Geometry: final body of the model. Coordinates: model frame, mm. Face numbers are marked on the shaded views. A direction names the side the tool comes from. Round coordinates to 2 decimals unless told otherwise and drop trailing zeros. Write each loop counter-clockwise with the first axis right and the second up, starting at its lowest first coordinate (ties: lowest second). Pieces come first, ordered by that corner, then holes. Notation, with made-up numbers: (-21, -39) -> (26, -39) arc R21 ccw to (26, -32) -> close; hole circle Ø5 at (19, 28). An arc over 180 degrees is marked (long way). Use one line per item in the form item = value. Start each with the question number.
1. Reachability of the marked faces 5, 6, 7 and 8 from +Z, -Z, +X, -X, +Y, -Y: full face, straight path, thin tool, end or side. Return the list, or none.
2. Cut plane B-B, the plane x = -29.5. Return the cut outline in (y, z).
3. Cut plane C-C, the plane z = 195. Return the cut outline in (x, y), plus the area to 3 significant figures.
4. Pin query (flat end, axial travel): pin 1 Ø10 at (x, z) = (12, 231) entering from +Y; pin 2 Ø4 at (x, z) = (33.5, 132.5) entering from +Y; pin 3 Ø25 at (y, z) = (-3, 237.5) entering from +X; pin 4 Ø10 at (x, y) = (-52.5, 21.5) entering from +Z. Return the tip coordinate at first contact, or that it passes through.
5. Cut plane D-D, the plane y = 54.5. Return the cut outline in (x, z), plus the area to 3 significant figures.
6. Line query: L1, parallel to X at y = 11, z = 203; L2, parallel to Y at x = 0, z = 138.5. Output: solid intervals per line, ascending.
7. Cut plane A-A, the plane y = 0. Return the cut outline in (x, z).
8. Draft query along Y for the marked faces 1, 2, 3 and 4. Return one class per face: pulls with the +Y half, pulls with the -Y half, needs draft (parallel to the pull), parting line crosses it, or undercut.
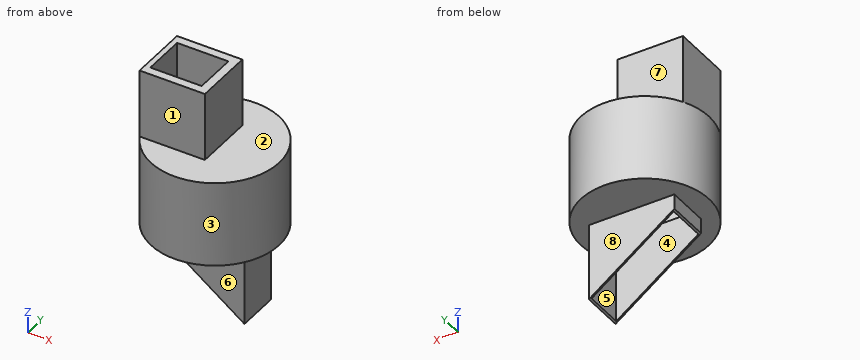
```python
from build123d import *

# Parameters (mm, degrees)
CROQUIS1_W              = 100
CROQUIS1_H              = 50
CROQUIS1_W_2            = 96
CROQUIS1_H_2            = 46
SALIENTE_EXTRUIR1_DEPTH = 100
CORTAR_EXTRUIR1_DEPTH   = 100
CROQUIS3_R              = 75
CROQUIS3_W              = 100
CROQUIS3_H              = 50
SALIENTE_EXTRUIR2_DEPTH = 10
SALIENTE_EXTRUIR3_START = 80
CROQUIS4_R              = 75
CROQUIS4_R_2            = 65
SALIENTE_EXTRUIR3_DEPTH = 80
SALIENTE_EXTRUIR4_START = 10
CROQUIS5_R              = 75
CROQUIS5_W              = 60
CROQUIS5_H              = 50
SALIENTE_EXTRUIR4_DEPTH = 10
CROQUIS6_W              = 76.332495807
CROQUIS6_H              = 70
CROQUIS6_W_2            = 60
CROQUIS6_H_2            = 50
SALIENTE_EXTRUIR5_DEPTH = 80


with BuildPart() as part:
    # Croquis1 → Saliente-Extruir1 (new body)
    with BuildSketch(Plane.XY):
        Rectangle(CROQUIS1_W, CROQUIS1_H)
        Rectangle(CROQUIS1_W_2, CROQUIS1_H_2, mode=Mode.SUBTRACT)
    extrude(amount=SALIENTE_EXTRUIR1_DEPTH)

    # Croquis2 → Cortar-Extruir1 (cut)
    with BuildSketch(Plane(origin=(0, 25, 0), x_dir=(1, 0, 0), z_dir=(0, 1, 0))):
        Polygon((-50, 0), (50, 0), (-50, -72.654252801), align=None)
    extrude(amount=-CORTAR_EXTRUIR1_DEPTH, mode=Mode.SUBTRACT)

    # Croquis3 → Saliente-Extruir2 (add)
    with BuildSketch(Plane.XY.offset(100)):
        Circle(CROQUIS3_R)
        Rectangle(CROQUIS3_W, CROQUIS3_H, mode=Mode.SUBTRACT)
    extrude(amount=-SALIENTE_EXTRUIR2_DEPTH)

    # Croquis4 → Saliente-Extruir3 (add)
    with BuildSketch(Plane.XY.offset(100).offset(SALIENTE_EXTRUIR3_START)):
        Circle(CROQUIS4_R)
        Circle(CROQUIS4_R_2, mode=Mode.SUBTRACT)
    extrude(amount=-SALIENTE_EXTRUIR3_DEPTH)

    # Croquis5 → Saliente-Extruir4 (add)
    with BuildSketch(Plane.XY.offset(180).offset(SALIENTE_EXTRUIR4_START)):
        Circle(CROQUIS5_R)
        with Locations((-30, 0)):
            Rectangle(CROQUIS5_W, CROQUIS5_H, mode=Mode.SUBTRACT)
    extrude(amount=-SALIENTE_EXTRUIR4_DEPTH)

    # Croquis6 → Saliente-Extruir5 (add)
    with BuildSketch(Plane.XY.offset(190)):
        with Locations((-28.166247904, 0)):
            Rectangle(CROQUIS6_W, CROQUIS6_H)
        with Locations((-30, 0)):
            Rectangle(CROQUIS6_W_2, CROQUIS6_H_2, mode=Mode.SUBTRACT)
    extrude(amount=SALIENTE_EXTRUIR5_DEPTH)


solid = part.part
```
Outcome:
q1.face_5 = -Z
q1.face_6 = -Z, +X, -X, -Y
q1.face_7 = +Z, +X, -X, +Y
q1.face_8 = -Z, +X, -X, +Y
q2.outline = (-68.95, 90) -> (-25, 90) -> (-25, 57.76) -> (-23, 57.76) -> (-23, 100) -> (-57.92, 100) -> (-57.92, 180) -> (-25, 180) -> (-25, 270) -> (-35, 270) -> (-35, 190) -> (-68.95, 190) -> close; (23, 57.76) -> (25, 57.76) -> (25, 90) -> (68.95, 90) -> (68.95, 190) -> (35, 190) -> (35, 270) -> (25, 270) -> (25, 180) -> (57.92, 180) -> (57.92, 100) -> (23, 100) -> close
q3.outline = (-66.33, -35) -> (10, -35) -> (10, 35) -> (-66.33, 35) -> close; hole (-60, -25) -> (0, -25) -> (0, 25) -> (-60, 25) -> close
q3.area = 2,340 mm^2
q4.pin_1 = 35
q4.pin_2 = 68.06
q4.pin_3 = 10
q4.pin_4 = 270
q5.outline = (-51.52, 90) -> (51.52, 90) -> (51.52, 190) -> (-51.52, 190) -> close; hole (-35.42, 100) -> (35.42, 100) -> (35.42, 180) -> (-35.42, 180) -> close
q5.area = 4,640 mm^2
q6.L1 = -66.33 to -60, 0 to 10
q6.L2 = -75 to -65, 65 to 75
q7.outline = (-75, 90) -> (-50, 90) -> (-50, 72.65) -> (-48, 71.2) -> (-48, 100) -> (-65, 100) -> (-65, 180) -> (-60, 180) -> (-60, 270) -> (-66.33, 270) -> (-66.33, 190) -> (-75, 190) -> close; (0, 180) -> (65, 180) -> (65, 100) -> (48, 100) -> (48, 1.45) -> (50, 0) -> (50, 90) -> (75, 90) -> (75, 190) -> (10, 190) -> (10, 270) -> (0, 270) -> close
q8.face_1 = pulls with the -Y half
q8.face_2 = needs draft
q8.face_3 = parting line crosses it
q8.face_4 = undercut
